Geometry: final body of the model. Coordinates: model frame, mm. Face numbers are marked on the shaded views. A direction names the side the tool comes from. Give positions to 0.01 mm unless a question says otherwise; leave off trailing zeros. Write each loop counter-clockwise with the first axis right and the second up, starting at its lowest first coordinate (ties: lowest second). Pieces come first, ordered by that corner, then holes. Notation, with made-up numbers: (-4.5, 40.5) - (20.5, 40.5) arc R12 ccw to (20.5, 47.5) - close; hole circle Ø7 at (-35, 86). An arc over 180 degrees is marked (long way). Use CSV: the item, a comma, the result in double quotes. Start each with the question number.
(1) Section A-A on x = -66. Output: boundary loops of the cut face in (y, z).
(2) Line query: probe 1 along Z at (x, y) = (-67.5, -3); probe 2 along X at (y, z) = (-14.5, -4); probe 3 along Z at (x, y) = (54, -10). Output: solid intervals per line, ascending. Write a range as [from, to].
(3) Draft query along Z for the marked faces 1 and 2. Return one class per face: released by +Z, released by -Z, zero draft, split by the parting line, or undercut.
(4) Reachability of the marked faces 3 and 4 from +Z, -Z, +X, -X, +Y, -Y: full face, straight path, thin tool, end or side. Return the list, or none.
(5) First-contact query: pin 1 Ø9.5 at (y, z) = (-11.5, -74.5) entering from -X; pin 2 Ø5 at (x, y) = (-37, -12) entering from +Z; pin 3 Ø10.5 at (x, y) = (-55, -5.5) entering from -Z; pin 4 Ø4 at (x, z) = (20, 25.5) entering from +Y. Flat tips, straight axial feed; report the tip coordinate or a pass-through.
from build123d import *

# Parameters (mm, degrees)
F1_DEPTH = 19.05


with BuildPart() as f1:
    # F0 (on Front) → F1 (new body)
    with BuildSketch(Plane.XZ):
        Polygon((80.9625, -65.0875), (80.9625, 65.0875), (71.4375, 65.0875), (71.4375, 84.1375), (61.9125, 84.1375), (61.9125, 65.0875), (52.3875, 65.0875), (52.3875, 84.1375), (42.8625, 84.1375), (42.8625, 65.0875), (33.3375, 65.0875), (33.3375, 84.1375), (23.8125, 84.1375), (23.8125, 65.0875), (14.2875, 65.0875), (14.2875, 84.1375), (4.7625, 84.1375), (4.7625, 65.0875), (-4.7625, 65.0875), (-4.7625, 84.1375), (-14.2875, 84.1375), (-14.2875, 65.0875), (-23.8125, 65.0875), (-23.8125, 83.364271), (-33.3375, 83.364271), (-33.3375, 65.0875), (-42.8625, 65.0875), (-42.8625, 82.642086), (-52.3875, 82.642086), (-52.3875, 65.0875), (-61.9125, 65.0875), (-61.9125, 83.017498), (-71.4375, 83.017498), (-71.4375, 65.0875), (-80.9625, 65.0875), (-80.9625, 12.7), (-61.9125, 12.7), (-61.9125, -12.7), (-80.9625, -12.7), (-80.9625, -65.0875), (-71.4375, -65.0875), (-71.4375, -83.017498), (-61.9125, -83.017498), (-61.9125, -65.0875), (-52.3875, -65.0875), (-52.3875, -82.642086), (-42.8625, -82.642086), (-42.8625, -65.0875), (-33.3375, -65.0875), (-33.3375, -83.364271), (-23.8125, -83.364271), (-23.8125, -65.0875), (-14.2875, -65.0875), (-14.2875, -84.1375), (-4.7625, -84.1375), (-4.7625, -65.0875), (4.7625, -65.0875), (4.7625, -84.1375), (14.2875, -84.1375), (14.2875, -65.0875), (23.8125, -65.0875), (23.8125, -84.1375), (33.3375, -84.1375), (33.3375, -65.0875), (42.8625, -65.0875), (42.8625, -84.1375), (52.3875, -84.1375), (52.3875, -65.0875), (61.9125, -65.0875), (61.9125, -84.1375), (71.4375, -84.1375), (71.4375, -65.0875), align=None)
    extrude(amount=F1_DEPTH)


solid = f1.part
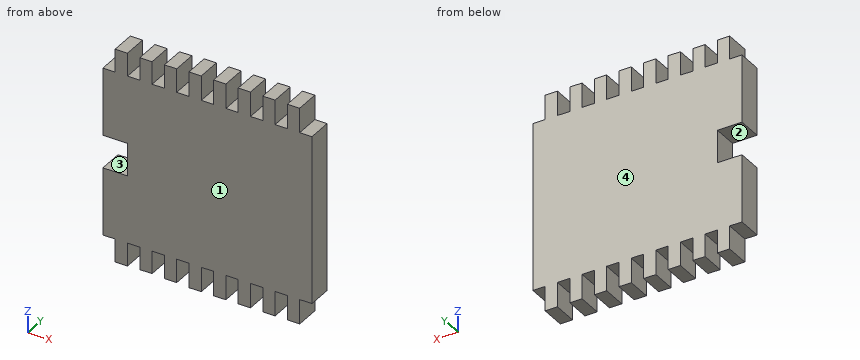
Check values:
1,outline,"(-19.05, -83.02) - (0, -83.02) - (0, -12.7) - (-19.05, -12.7) - close; (-19.05, 12.7) - (0, 12.7) - (0, 83.02) - (-19.05, 83.02) - close"
2,probe 1,"z = [-83.02, -12.7], [12.7, 83.02]"
2,probe 2,"x = [-61.91, 80.96]"
2,probe 3,"z = [-65.09, 65.09]"
3,face 1,"zero draft"
3,face 2,"undercut"
4,face 3,"-X, +Y, -Y"
4,face 4,"+Z, -Z, +X, -X, +Y"
5,pin 1,"stops at x = -71.44"
5,pin 2,"stops at z = 65.09"
5,pin 3,"stops at z = -82.64"
5,pin 4,"stops at y = 0"
